from build123d import *

# Parameters (mm, degrees)
CROQUIS1_W              = 60.2
CROQUIS1_H              = 14
SALIENTE_EXTRUIR1_DEPTH = 30
CROQUIS2_W              = 12
CROQUIS2_H              = 25.4
CORTAR_EXTRUIR1_DEPTH   = 14
CORTAR_EXTRUIR2_START   = -30
CROQUIS3_W              = 12.5
CROQUIS3_H              = 7
CROQUIS3_W_2            = 10
CORTAR_EXTRUIR2_DEPTH   = 30
CORTAR_EXTRUIR3_DEPTH   = 21
CROQUIS5_W              = 12
CROQUIS5_H              = 4
CORTAR_EXTRUIR4_DEPTH   = 3.3
SALIENTE_EXTRUIR2_DEPTH = 3
SALIENTE_EXTRUIR3_DEPTH = 3


with BuildPart() as part:
    # Croquis1 → Saliente-Extruir1 (new body)
    with BuildSketch(Plane(origin=(0, 0, 0), x_dir=(1, 0, 0), z_dir=(0, 1, 0))):
        with Locations((-26.023666378, 13.176470588)):
            Rectangle(CROQUIS1_W, CROQUIS1_H)
    extrude(amount=SALIENTE_EXTRUIR1_DEPTH)

    # Croquis2 → Cortar-Extruir1 (cut)
    with BuildSketch(Plane.XY.offset(-6.176470588)):
        Polygon((-48.123666378, 0), (-18.423666378, 0), (-18.423666378, 4), (-14.423666378, 4), (-14.423666378, 5.7), (-19.023666378, 5.7), (-50.023666378, 5.7), (-52.123666378, 5.7), (-52.123666378, 4), (-48.123666378, 4), align=None)
        with Locations((-5.923666378, 17.3)):
            Rectangle(CROQUIS2_W, CROQUIS2_H)
    extrude(amount=-CORTAR_EXTRUIR1_DEPTH, mode=Mode.SUBTRACT)

    # Croquis3 → Cortar-Extruir2 (cut)
    with BuildSketch(Plane(origin=(0, 30, 0), x_dir=(1, 0, 0), z_dir=(0, 1, 0)).offset(CORTAR_EXTRUIR2_START)):
        with Locations((-49.873666378, 13.676470588)):
            Rectangle(CROQUIS3_W, CROQUIS3_H)
        with Locations((-16.923666378, 13.676470588)):
            Rectangle(CROQUIS3_W_2, CROQUIS3_H)
    extrude(amount=CORTAR_EXTRUIR2_DEPTH, mode=Mode.SUBTRACT)

    # Croquis4 → Cortar-Extruir3 (cut)
    with BuildSketch(Plane(origin=(0, 30, 0), x_dir=(1, 0, 0), z_dir=(0, 1, 0))):
        Polygon((-43.623666378, 17.176470588), (-21.923666378, 17.176470588), (-21.923666378, 10.176470588), (-16.923666378, 10.176470588), (-16.923666378, 6.176470588), (-56.123666378, 6.176470588), (-56.123666378, 10.176470588), (-43.623666378, 10.176470588), align=None)
    extrude(amount=-CORTAR_EXTRUIR3_DEPTH, mode=Mode.SUBTRACT)

    # Croquis5 → Cortar-Extruir4 (cut)
    with BuildSketch(Plane(origin=(0, 9, 0), x_dir=(1, 0, 0), z_dir=(0, 1, 0))):
        with Locations((-31.523666378, 8.176470588)):
            Rectangle(CROQUIS5_W, CROQUIS5_H)
    extrude(amount=-CORTAR_EXTRUIR4_DEPTH, mode=Mode.SUBTRACT)

    # Croquis6 → Saliente-Extruir2 (add)
    with BuildSketch(Plane.XY.offset(-6.176470588)):
        Polygon((-14.423666378, 5.7), (-11.923666378, 5.7), (-11.923666378, 4.6), (0.076333622, 4.6), (0, 0), (-14.423666378, 0), align=None)
    extrude(amount=SALIENTE_EXTRUIR2_DEPTH)

    # Croquis7 → Saliente-Extruir3 (add)
    with BuildSketch(Plane(origin=(0, 0, -20.176470588), x_dir=(-1, 0, 0), z_dir=(0, 0, -1))):
        Polygon((14.423666378, 5.7), (11.923666378, 5.7), (11.923666378, 4.6), (-0.076333622, 4.6), (0, 0), (14.423666378, 0), align=None)
    extrude(amount=SALIENTE_EXTRUIR3_DEPTH)


solid = part.part
Read the model definition and answer for the solid it produces. Units are mm, in the model's axes. A direction names the side the tool comes from. Round coordinates to 2 decimals unless told otherwise and drop trailing zeros. Loops run counter-clockwise (first coordinate to the right, second up) from the corner with the lowest first, then second, coordinate; pieces in that order, holes last.
Q1. Section B-B on x = -49 is taken. Write down the section's boundary in (y, z).
Q2. Each of these flat-tipped pins is pushed along its axis until it touches: pin 1 (10 mm diameter, centred on x = -27, z = -11.5, fed in from +Y); pin 2 (1.5 mm diameter, centred on x = -15, y = 7, fed in from +Z); pin 3 (10 mm diameter, centred on x = -37, z = -20, fed in from -Y); pin 4 (4.5 mm diameter, centred on x = -45.5, y = 2.5, fed in from +Z). Where does it stop, or does it pass through?
Q3. Which of the six approach directions +Z, -Z, +X, -X, +Y, -Y give full straight-line access (tool end or side, diameter ignored) to faces 4 (the face through (-49, 6, -6.176)), 5 (the face through (-50, 4, -19)), 6 (the face through (-14.424, 3, -6)), 7 (the face through (-16.924, 20, -8)), 8 (the face through (-43.624, 7, -14))?
Q4. Determine the mould class of faces 1 (the face through (-11.924, 17, -19)), 2 (the face through (-14.424, 3, -21)), 3 (the face through (-52, 0, -8)) for opening direction Y: released by +Y, released by -Y, zero draft, split by the parting line, or undercut.
Q5. Section C-C on y = 25.5 is taken. Write down the section's boundary in (x, z), and give its area (3 significant figures).
Q6. Section D-D on z = -18.25 is taken. Write down the section's boundary in (x, y), and give its area (3 significant figures).
Q7. Section A-A on z = -9 is taken. Write down the section's boundary in (x, y).
Q8. Consider probe 1 along Z at (x, y) = (-12, 28); probe 2 along Z at (x, y) = (-13.5, 2); probe 3 along X at (y, z) = (9.5, -17.25). Determine where each line is inside the solid, lowest interval first.
Output:
1. outline: (0, -20.18) - (4, -20.18) - (4, -17.18) - (0, -17.18) - close; (0, -10.18) - (4, -10.18) - (4, -6.18) - (0, -6.18) - close; (5.7, -20.18) - (30, -20.18) - (30, -17.18) - (5.7, -17.18) - close; (5.7, -10.18) - (9, -10.18) - (9, -6.18) - (5.7, -6.18) - close
2. pin 1: stops at y = 9
2. pin 2: stops at z = -6.18
2. pin 3: stops at y = 5.7
2. pin 4: passes through
3. face 4: +Z, -X, +Y, -Y
3. face 5: +Z, -Z
3. face 6: +Z
3. face 7: +Z, -X, +Y
3. face 8: -X, +Y, -Y
4. face 1: zero draft
4. face 2: undercut
4. face 3: released by -Y
5. outline: (-56.12, -20.18) - (-11.92, -20.18) - (-11.92, -17.18) - (-56.12, -17.18) - close; (-16.92, -10.18) - (-11.92, -10.18) - (-11.92, -6.18) - (-16.92, -6.18) - close; (0.08, -20.18) - (4.08, -20.18) - (4.08, -6.18) - (0.08, -6.18) - close
5. area: 209 mm2
6. outline: (-56.12, 0) - (-48.12, 0) - (-48.12, 4) - (-52.12, 4) - (-52.12, 5.7) - (-14.42, 5.7) - (-14.42, 4) - (-18.42, 4) - (-18.42, 0) - (4.08, 0) - (4.08, 30) - (0.08, 30) - (0.08, 4.6) - (-11.92, 4.6) - (-11.92, 30) - (-56.12, 30) - close
6. area: 1,320 mm2
7. outline: (-56.12, 0) - (-48.12, 0) - (-48.12, 4) - (-52.12, 4) - (-52.12, 5.7) - (-37.52, 5.7) - (-37.52, 9) - (-56.12, 9) - close; (-25.52, 5.7) - (-14.42, 5.7) - (-14.42, 4) - (-18.42, 4) - (-18.42, 0) - (4.08, 0) - (4.08, 30) - (0.08, 30) - (0.08, 4.6) - (-11.92, 4.6) - (-11.92, 30) - (-16.92, 30) - (-16.92, 9) - (-25.52, 9) - close
8. probe 1: z = -20.18 to -17.18, -10.18 to -6.18
8. probe 2: z = -23.18 to -17.18, -10.18 to -3.18
8. probe 3: x = -56.12 to -11.92, 0.08 to 4.08
